Can you work these out from the drawing? Everything is in mm from the part's minimum corner. Give positions to 0.01 mm unless a question says otherwise; leave off trailing zeros. Loops run counter-clockwise (first coordinate to the right, second up) from the corner with the lowest first, then second, coordinate; pieces in that order, holes last. Notation, with made-up numbers: (4.5, -34) - (29.5, -34) arc R30 ccw to (29.5, 1) - close; hole circle Ø1 at (-38, 7). An arc over 180 degrees is marked (long way). One line per item, written item: value. Start each with the question number.
Q1. I'm going to push a flat-ended pin straight in: P1, Ø1.8, axis at x = 3.46, y = 3, coming from the -Z side. Where does the tip first touch, or does it pass through?
Q2. I want a section at A-A (z = 1.05). Please give me the cut outline in (x, y) (1 decimal), then the cut area to 3 significant figures.
Q3. If we mould it in two halves opening along Y, with no side actions, what happens to the marked faces 1, 2 and 3? For each: released by +Y, released by -Y, zero draft, split by the parting line, or undercut.
Q4. I want a section at B-B (z = 0.4). Please give me the cut outline in (x, y) (1 decimal).
Q5. If I drill on line 1 (Y direction, x = 3.5, z = 0.9); line 2 (X direction, y = 4.25, z = 0.85) (1 decimal); line 3 (Y direction, x = 2.5, z = 0.6), over which ranges is the centre line in solid material (lowest first)? Write a range as from..to.
Q6. I want a section at C-C (z = 1.6). Please give me the cut outline in (x, y) (1 decimal).
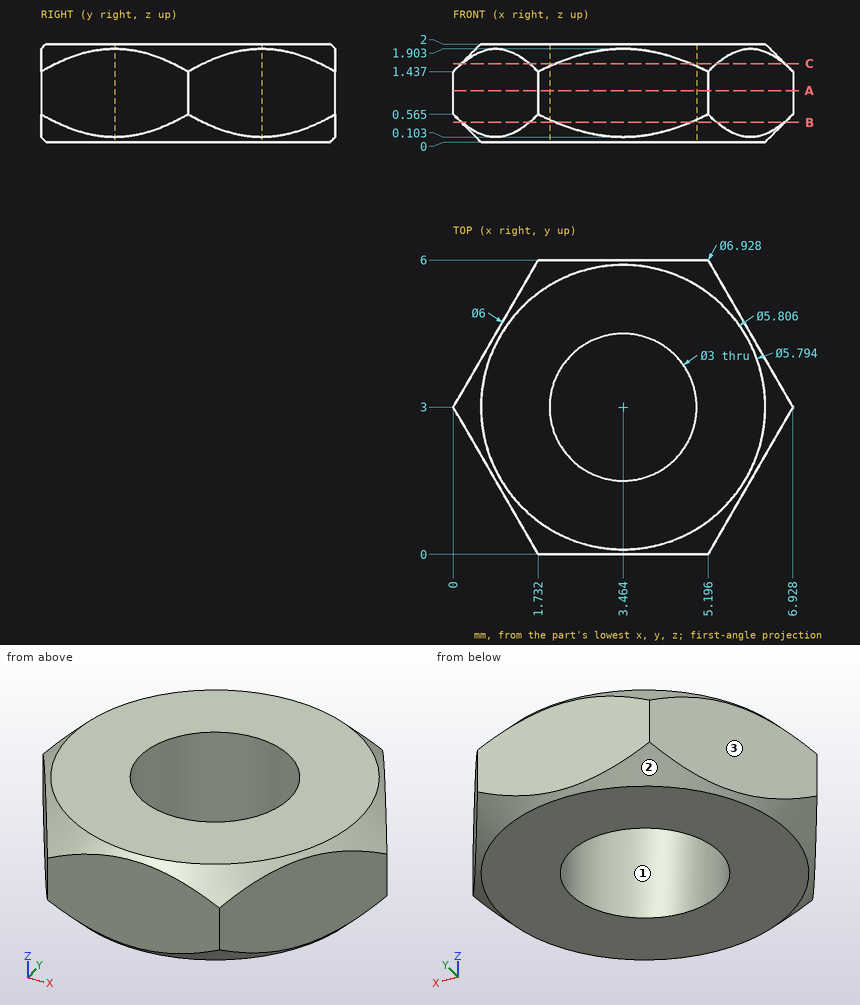
Worked answers:
1. P1: passes through
2. outline: (0, 3) - (1.7, 0) - (5.2, 0) - (6.9, 3) - (5.2, 6) - (1.7, 6) - close; hole circle Ø3 at (3.5, 3)
2. area: 24.1 mm²
3. face 1: undercut
3. face 2: split by the parting line
3. face 3: released by +Y
4. outline: (0.2, 2.7) - (1.6, 0.3) arc R3.3 ccw to (2.1, 0) - (4.8, 0) arc R3.3 ccw to (5.4, 0.3) - (6.7, 2.7) arc R3.3 ccw to (6.7, 3.3) - (5.4, 5.7) arc R3.3 ccw to (4.8, 6) - (2.1, 6) arc R3.3 ccw to (1.6, 5.7) - (0.2, 3.3) arc R3.3 ccw to start; hole circle Ø3 at (3.5, 3)
5. line 1: y = 0..1.5, 4.5..6
5. line 2: x = 0.7..2.6, 4.3..6.2
5. line 3: y = 0..1.85, 4.15..6
6. outline: (0.2, 2.7) - (1.6, 0.3) arc R3.3 ccw to (2.1, 0) - (4.8, 0) arc R3.3 ccw to (5.4, 0.3) - (6.8, 2.7) arc R3.3 ccw to (6.8, 3.3) - (5.4, 5.7) arc R3.3 ccw to (4.8, 6) - (2.1, 6) arc R3.3 ccw to (1.6, 5.7) - (0.2, 3.3) arc R3.3 ccw to start; hole circle Ø3 at (3.5, 3)
